Could you check a few things on this model? Use its own coordinates, in mm. A direction names the side the tool comes from. Give positions to 0.01 mm unless a question says otherwise; leave off trailing zeros. Loops run counter-clockwise (first coordinate to the right, second up) from the corner with the lowest first, then second, coordinate; pieces in that order, holes last. Notation, with made-up numbers: M -26.75,-36 L -4.75,-36 A23 ccw -4.75,-27 Z; hole C 83,-31 d4. An arc over 180 degrees is marked long. Answer in a Markdown table with one row per item. Add a question column.
1. I'm going to push flat-ended pins straight in: pin 1 Ø4 at (x, y) = (-188.71, -100) entering from +Z; pin 2 Ø5 at (x, z) = (-138, 19) entering from +Y; pin 3 Ø1.5 at (y, z) = (-95.5, 24.5) entering from -X. Where does each tip first touch, or does it pass through?
2. I need wall thicknesses on line 1 along Y through (x, z) = (-29, 6.5); line 2 along Y through (x, z) = (-5, 23); line 3 along Y through (x, z) = (-14.5, 33.5). Which ranges of each line are inside material? Lowest first, please. Write a range as from..to.
3. Which directions (+Z, -Z, +X, -X, +Y, -Y) give clear straight access to the entire face, cutting with the end or side of a thin tool? Please do faces 4 (the cylindrical face through (-27.95, -5.06, 20.78)), 5 (the flat face through (-14, -200, 18)).
4. Thinking about a two-plate mould opening in X: for faces 1 (the flat face through (-110.924, -147.794, 20.776)), 2 (the flat face through (2.5, -101, 18)), 3 (the flat face through (-14, 0, 18)), which applies, released by +X, released by -X, zero draft, split by the parting line, or undercut?
5. If we section it at D-D on x = -156.5: List the corners of the cut face in (y, z) for me, then the cut area to 3 significant figures.
6. If we section it at B-B on x = -5: List the corners of the cut face in (y, z) for me.
7. If we section it at A-A on z = 12: List the corners of the cut face in (x, y) for me, then the cut area to 3 significant figures.
8. If we section it at C-C on y = -113.5: List the corners of the cut face in (x, z) for me, then the cut area to 3 significant figures.
```python
from build123d import *

# Parameters (mm, degrees)
BOSS_EXTRUDE1_DEPTH = 5
SKETCH2_R           = 2.5
BOSS_EXTRUDE2_DEPTH = 32


with BuildPart() as part:
    # Sketch1 → Boss-Extrude1 (new body)
    with BuildSketch(Plane.XY):
        Polygon((-30.5, -200), (-203.705080757, -100), (-30.5, 0), (2.5, 0), (2.5, -200), align=None)
    extrude(amount=BOSS_EXTRUDE1_DEPTH)

    # Sketch2 → Boss-Extrude2 (add)
    with BuildSketch(Plane.XY.offset(5)):
        Polygon((-203.705080757, -100), (-30.5, -200), (2.5, -200), (2.5, 0), (-30.5, 0), align=None)
        with Locations((-188.705080757, -100)):
            Circle(SKETCH2_R, mode=Mode.SUBTRACT)
        with Locations((-5, -192.5)):
            Circle(SKETCH2_R, mode=Mode.SUBTRACT)
        with Locations(Location((-5, -7.5, 0), (0, 0, 180))):
            Circle(SKETCH2_R, mode=Mode.SUBTRACT)
        with Locations((-28.490381057, -192.5)):
            Circle(SKETCH2_R, mode=Mode.SUBTRACT)
        with Locations(Location((-28.490381057, -7.5, 0), (0, 0, 180))):
            Circle(SKETCH2_R, mode=Mode.SUBTRACT)
        with BuildLine():
            Line((-8.741657387, -5), (-24.74872367, -5))
            ThreePointArc((-24.74872367, -5), (-27.325695354, -11.846666218), (-32.980751406, -7.205765184))
            Line((-32.980751406, -7.205765184), (-186.714710408, -95.964107797))
            ThreePointArc((-186.714710408, -95.964107797), (-184.205080757, -100), (-186.714710408, -104.035892203))
            Line((-186.714710408, -104.035892203), (-32.980751406, -192.794234816))
            ThreePointArc((-32.980751406, -192.794234816), (-27.325695354, -188.153333782), (-24.74872367, -195))
            Line((-24.74872367, -195), (-8.741657387, -195))
            ThreePointArc((-8.741657387, -195), (-8.181980515, -189.318019485), (-2.5, -188.758342613))
            Line((-2.5, -188.758342613), (-2.5, -11.241657387))
            ThreePointArc((-2.5, -11.241657387), (-8.181980515, -10.681980515), (-8.741657387, -5))
        make_face(mode=Mode.SUBTRACT)
    extrude(amount=BOSS_EXTRUDE2_DEPTH)


solid = part.part
```
Results:
| question | item | result |
|---|---|---|
| 1 | pin 1 | z = 5 |
| 1 | pin 2 | y = -60.62 |
| 1 | pin 3 | x = -197.21 |
| 2 | line 1 | -200..-194.95, -190.05..-188.03, -11.97..-9.95, -5.05..0 |
| 2 | line 2 | -200..-195, -190..-188, -12..-10, -5..0 |
| 2 | line 3 | -200..-195, -5..0 |
| 3 | face 4 | +Z |
| 3 | face 5 | +Z, -Z, +X, -X, -Y |
| 4 | face 1 | undercut |
| 4 | face 2 | released by +X |
| 4 | face 3 | zero draft |
| 5 | outline | M -127.25,0 L -72.75,0 L -72.75,37 L -78.52,37 L -78.52,5 L -121.48,5 L -121.48,37 L -127.25,37 Z |
| 5 | area | 642 mm2 |
| 6 | outline | M -200,0 L 0,0 L 0,37 L -5,37 L -5,5 L -10,5 L -10,37 L -12,37 L -12,5 L -188,5 L -188,37 L -190,37 L -190,5 L -195,5 L -195,37 L -200,37 Z |
| 7 | outline | M -203.71,-100 L -30.5,-200 L 2.5,-200 L 2.5,0 L -30.5,0 Z; hole C -188.71,-100 d5; hole M -186.71,-104.04 L -32.98,-192.79 A4.5 cw long -24.75,-195 L -8.74,-195 A4.5 cw -2.5,-188.76 L -2.5,-11.24 A4.5 cw -8.74,-5 L -24.75,-5 A4.5 cw long -32.98,-7.21 L -186.71,-95.96 A4.5 cw Z; hole C -28.49,-192.5 d5; hole C -28.49,-7.5 d5; hole C -5,-192.5 d5; hole C -5,-7.5 d5 |
| 7 | area | 3,350 mm2 |
| 8 | outline | M -180.32,0 L 2.5,0 L 2.5,37 L -2.5,37 L -2.5,5 L -170.32,5 L -170.32,37 L -180.32,37 Z |
| 8 | area | 1,390 mm2 |
